Autodesk Inventor part; units mm, degrees
ref_plane "YZ Plane" through (0, 0, 0) normal (1, 0, 0) x (0, 1, 0)
ref_plane "XZ Plane" through (0, 0, 0) normal (0, 1, 0) x (-1, 0, 0)
ref_plane "XY Plane" through (0, 0, 0) normal (0, 0, 1) x (1, 0, 0)
sketch "Sketch34" plane through (0, 0, 0) normal (0, 0, 1) x (1, 0, 0)
  line L0 (0, 0) -> (30, 0)
  line L1 (30, 0) -> (30, -30)
  line L2 (30, -30) -> (0, -30)
  line L3 (0, -30) -> (0, 0)
  dimension "d112" = 30
  dimension "d113" = 30
extrude "Extrusion25" add sketch "Sketch34" against normal blind 10
sketch "Sketch35" plane through (30, -30, 0) normal (1, 0, 0) x (0, 0, -1)
  line L0 (0, 30) -> (10, 30)
  line L1 (0, 30) -> (30, 30)
  line L2 (30, 30) -> (30, 0)
  line L3 (30, 0) -> (0, 0)
  line L4 (0, 0) -> (0, 30)
  dimension "d116" = 30
  dimension "d117" = 30
extrude "Extrusion26" add sketch "Sketch35" against normal blind 10
sketch "Sketch36" plane through (0, 0, 0) normal (0, 0, 1) x (1, 0, 0)
  circle A0 centre (15, -15) radius 2.5
  point P0 (0, 0)
  dimension "d120" = 5
extrude "Extrusion27" cut sketch "Sketch36" against normal blind 10
sketch "Sketch37" plane through (30, -30, 0) normal (1, 0, 0) x (0, 0, -1)
  point P0 (0, 30)
sketch "Sketch38" plane through (30, -30, 0) normal (1, 0, 0) x (0, 0, -1)
  circle A0 centre (15, 15) radius 2.5
  point P0 (0, 30)
  dimension "d123" = 5
extrude "Extrusion28" cut sketch "Sketch38" against normal blind 10
sketch "Sketch39" plane through (30, -30, 0) normal (1, 0, 0) x (0, 0, -1)
  point P0 (0, 30)
sketch "Sketch42" plane through (0, 0, -10) normal (0, 0, -1) x (-1, 0, 0)
  circle A0 centre (-15, -15) radius 4
  point P0 (0, 0)
  dimension "d132" = 8
extrude "Extrusion31" cut sketch "Sketch42" against normal blind 5
sketch "Sketch43" plane through (20, -30, 0) normal (-1, 0, 0) x (0, 0, 1)
  circle A0 centre (-15, 15) radius 4
  point P0 (0, 30)
  dimension "d135" = 8
extrude "Extrusion32" cut sketch "Sketch43" against normal blind 5
properties part number "tunnel corner bracket"
Can you work these out from the model? Positions are in its coordinate system, mm. A direction names the side the tool comes from. Give positions to 0.01 mm unless a question says otherwise; leave off trailing zeros. Order: outer loops, then holes, each group sorted by start corner. A loop starts at its lowest first (then second) coordinate and runs counter-clockwise, first axis right, second up. Notation, with made-up numbers: M 6,-5.5 L 22,-5.5 A19 ccw 22,12.5 Z; hole C 22.5,46.5 d6. An arc over 180 degrees is marked long. Use one line per item in the form item = value.
Item 1: Thinking about a two-plate mould opening in Y: for faces 4 (the flat face through (25, -17, -17)), 5 (the flat face through (19, -30, -8)), 6 (the cylindrical face through (27.5, -14.9, -12.5)), 7 (the flat face through (0, -15, -5)), which applies, pulls with the +Y half, pulls with the -Y half, needs draft (parallel to the pull), parting line crosses it, or undercut?
Values follow:
face_4 = undercut
face_5 = pulls with the -Y half
face_6 = undercut
face_7 = needs draft
Item 2: Will these pins go through, and if not, where does the flat tip stop? pin 1 Ø3 at (y, z) = (-15, -15) entering from +X; pin 2 Ø1.5 at (x, y) = (5, -18.5) entering from -Z; pin 3 Ø2 at (y, z) = (-7, -11.5) entering from -X; pin 4 Ø2.5 at (y, z) = (-16, -16.5) entering from -X.
Values follow:
pin_1 = through
pin_2 = -10
pin_3 = 20
pin_4 = 25
Item 3: If we section it at C-C, the plane z = -15: Write out the boundary of the cut face in (x, y), and give its area (3 significant figures).
Values follow:
outline = M 20,-30 L 30,-30 L 30,-17.5 L 25,-17.5 L 25,-19 L 20,-19 Z; M 20,-11 L 25,-11 L 25,-12.5 L 30,-12.5 L 30,0 L 20,0 Z
area = 235 mm^2
Item 4: If we section it at A-A, the plane y = -15: Write out the boundary of the cut face in (x, z), and give its area (3 significant figures).
Values follow:
outline = M 0,-10 L 11,-10 L 11,-5 L 12.5,-5 L 12.5,0 L 0,0 Z; M 17.5,-5 L 19,-5 L 19,-10 L 20,-10 L 20,-11 L 25,-11 L 25,-12.5 L 30,-12.5 L 30,0 L 17.5,0 Z; M 20,-30 L 30,-30 L 30,-17.5 L 25,-17.5 L 25,-19 L 20,-19 Z
area = 370 mm^2
Item 5: If we section it at B-B, the plane x = 15: Write out the boundary of the cut face in (y, z), and give its area (3 significant figures).
Values follow:
outline = M -30,-10 L -19,-10 L -19,-5 L -17.5,-5 L -17.5,0 L -30,0 Z; M -12.5,-5 L -11,-5 L -11,-10 L 0,-10 L 0,0 L -12.5,0 Z
area = 235 mm^2
Item 6: If we section it at D-D, the plane z = -4.5: Write out the boundary of the cut face in (x, y).
Values follow:
outline = M 0,-30 L 30,-30 L 30,0 L 0,0 Z; hole C 15,-15 d5
Item 7: If I drill on line 1 along Y through (x, z) = (27.1, -15); line 2 along Y through (x, z) = (23.2, -15); line 3 along Z through (x, y) = (6.5, -8.5), over which ranges is the centre line in solid material (lowest first)? Write a range as [from, to].
Values follow:
line_1 = [-30, -17.5], [-12.5, 0]
line_2 = [-30, -19], [-11, 0]
line_3 = [-10, 0]
Item 8: For faces 1 (the flat face through (20, -15, -20)), 2 (the cylindrical face through (22, -15, -19)), 3 (the flat face through (17, -17, -5)), which set-ups out of +Z, -Z, +X, -X, +Y, -Y let a thin tool reach every point of the face, with its end or its side?
Values follow:
face_1 = -Z, -X, +Y, -Y
face_2 = -X
face_3 = -Z
